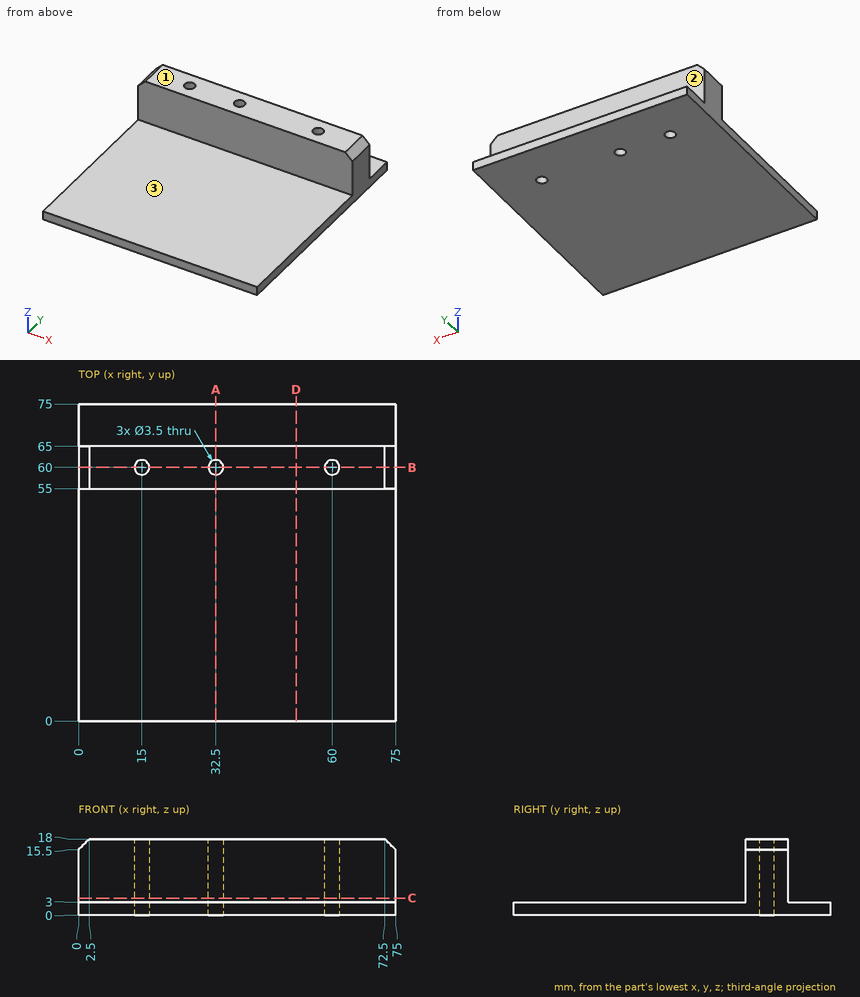
Input: dimensioned drawing with shaded views. Units: mm. Origin: part minimum x, y, z. A direction names the side the tool comes from. Give positions to 0.01 mm unless a question says otherwise; leave off trailing zeros. Write each loop counter-clockwise with the first axis right and the second up, starting at its lowest first coordinate (ties: lowest second). Pieces come first, ordered by that corner, then holes. Notation, with made-up numbers: (-14.5, 45) -> (-5.5, 45) arc R29 ccw to (-5.5, 77) -> close; hole circle Ø7 at (12.5, -23.5). An arc over 180 degrees is marked (long way). Return JSON: item names as keys, results as strings. Group by question number.
1. Access query for the marked faces 1, 2 and 3. Directions: +Z, -Z, +X, -X, +Y, -Y. A direction counts if a zero-diameter tool reaches every point of the face in a straight line with its end or side. Return the directions, or none.
2. Section C-C, the plane z = 4. Output: boundary loops of the cut face in (x, y), then the cut area to 3 significant figures.
3. Section D-D, the plane x = 51.5. Output: boundary loops of the cut face in (y, z), then the cut area to 3 significant figures.
4. Section B-B, the plane y = 60. Output: boundary loops of the cut face in (x, z), then the cut area to 3 significant figures.
5. Section A-A, the plane x = 32.5. Output: boundary loops of the cut face in (y, z), then the cut area to 3 significant figures.
6. Pin query (flat end, axial travel): pin 1 Ø3 at (x, z) = (34, 7.5) entering from +Y; pin 2 Ø1.5 at (x, z) = (19.5, 11) entering from -Y; pin 3 Ø2 at (x, y) = (60, 60) entering from +Z; pin 4 Ø10 at (x, y) = (33, 22) entering from +Z. Return the tip coordinate at first contact, or that it passes through.
7. Material intervals for line 1 (Y direction, x = 60, z = 8); line 2 (Y direction, x = 8, z = 10.75); line 3 (Y direction, x = 31, z = 7.5), sorted ascending. Write a range as from..to.
Determined:
{
 "1": {"face 1": "+Z, +X, -X, +Y, -Y", "face 2": "+Z, +X, -X, +Y", "face 3": "+Z, +X, -X, -Y"},
 "2": {"outline": "(0, 55) -> (75, 55) -> (75, 65) -> (0, 65) -> close; hole circle Ø3.5 at (15, 60); hole circle Ø3.5 at (32.5, 60); hole circle Ø3.5 at (60, 60)", "area": "721 mm2"},
 "3": {"outline": "(0, 0) -> (75, 0) -> (75, 3) -> (65, 3) -> (65, 18) -> (55, 18) -> (55, 3) -> (0, 3) -> close", "area": "375 mm2"},
 "4": {"outline": "(0, 0) -> (13.25, 0) -> (13.25, 18) -> (2.5, 18) -> (0, 15.5) -> close; (16.75, 0) -> (30.75, 0) -> (30.75, 18) -> (16.75, 18) -> close; (34.25, 0) -> (58.25, 0) -> (58.25, 18) -> (34.25, 18) -> close; (61.75, 0) -> (75, 0) -> (75, 15.5) -> (72.5, 18) -> (61.75, 18) -> close", "area": "1,150 mm2"},
 "5": {"outline": "(0, 0) -> (58.25, 0) -> (58.25, 18) -> (55, 18) -> (55, 3) -> (0, 3) -> close; (61.75, 0) -> (75, 0) -> (75, 3) -> (65, 3) -> (65, 18) -> (61.75, 18) -> close", "area": "312 mm2"},
 "6": {"pin 1": "stops at y = 65", "pin 2": "stops at y = 55", "pin 3": "passes through", "pin 4": "stops at z = 3"},
 "7": {"line 1": "y = 55..58.25, 61.75..65", "line 2": "y = 55..65", "line 3": "y = 55..59.1, 60.9..65"}
}
